```python
from build123d import *

# Parameters (mm, degrees)
F0_W      = 13
F0_H      = 7
F0_H_2    = 30.8050829545
F0_H_3    = 4
F1_DEPTH  = 13
F3_R      = 1.99999
F4_R      = 0.99999
F5_D      = 2.2
F7_W      = 3
F7_H      = 6.5
F6_W      = 66.7
F6_H      = 6.5
F8_DEPTH  = 2
F9_DEPTH  = 2
F10_R     = 3.5
F10_R_2   = 1.1
F11_DEPTH = 0.75


# Not quite as in the source:
# - a fillet or chamfer is up to 0.001 mm smaller than in the source, because OpenCascade refuses the exact size


with BuildPart() as f1:
    # F0 (on Top) → F1 (new body)
    with BuildSketch(Plane.XY):
        Polygon((-22, 0), (0, 0), (0, 3), (-19.5, 3), (-19.5, 5.3), (0, 5.3), (0, 72), (-15.5, 72), (-15.5, 100), (-20, 100), (-20, 62), (-18, 62), (-18, 59), (-20, 59), (-20, 22.1949170455), (-18, 22.1949170455), (-18, 19.1949170455), (-20, 19.1949170455), (-20, 9.1949170455), (-22, 9.1949170455), align=None)
        with Locations((-11.5, 12.6949170455)):
            Rectangle(F0_W, F0_H, mode=Mode.SUBTRACT)
        with Locations((-11.5, 40.5974585228)):
            Rectangle(F0_W, F0_H_2, mode=Mode.SUBTRACT)
        with Locations((-11.5, 67)):
            Rectangle(F0_W, F0_H_3, mode=Mode.SUBTRACT)
    extrude(amount=F1_DEPTH)

    # F3 (radius 2 in the source; OpenCascade refuses exactly that, so slightly less here)
    f3_edges = [f1.edges().sort_by_distance(p)[0] for p in [
        (-22, 0, 6.5),
        (-18, 69, 6.5),
        (-18, 65, 6.5),
        (-5, 69, 6.5),
        (-5, 65, 6.5),
        (-18, 56, 6.5),
        (-5, 56, 6.5),
        (-18, 25.194917, 6.5),
        (-5, 25.194917, 6.5),
        (-18, 9.194917, 6.5),
        (-5, 9.194917, 6.5),
        (-5, 16.194917, 6.5),
        (-18, 16.194917, 6.5),
    ]]
    fillet(f3_edges, radius=F3_R)

    # F4 (radius 1 in the source; OpenCascade refuses exactly that, so slightly less here)
    f4_edges = [f1.edges().sort_by_distance(p)[0] for p in [
        (-15.5, 72, 6.5),
        (-20, 100, 6.5),
        (-22, 9.194917, 6.5),
        (-20, 9.194917, 6.5),
    ]]
    fillet(f4_edges, radius=F4_R)

    # F5 (through all)
    with Locations(Plane(origin=(-20, 0, 0), x_dir=(0, -1, 0), z_dir=(-1, 0, 0))):
        with Locations((-90, 6.5)):
            Hole(F5_D / 2)

    # F7 (on face) + F6 (on face) → F8 (join)
    with BuildSketch(Plane.YZ):
        with Locations((1.5, 3.25)):
            Rectangle(F7_W, F7_H)
    with BuildSketch(Plane.YZ):
        with Locations((38.65, 3.25)):
            Rectangle(F6_W, F6_H)
    extrude(amount=F8_DEPTH)

    # F9 (cut): faces of the model
    f9_faces = [f1.faces().sort_by_distance(p)[0] for p in [
        (0, 1.5, 9.75),
        (0, 38.65, 9.75),
    ]]
    extrude(f9_faces, amount=-F9_DEPTH, mode=Mode.SUBTRACT)

    # F10 (on face) → F11 (cut)
    with BuildSketch(Plane.YZ.offset(-15.5)):
        with Locations((90, 6.5)):
            Circle(F10_R)
        with Locations((90, 6.5)):
            Circle(F10_R_2, mode=Mode.SUBTRACT)
    extrude(amount=-F11_DEPTH, mode=Mode.SUBTRACT)


solid = f1.part
```
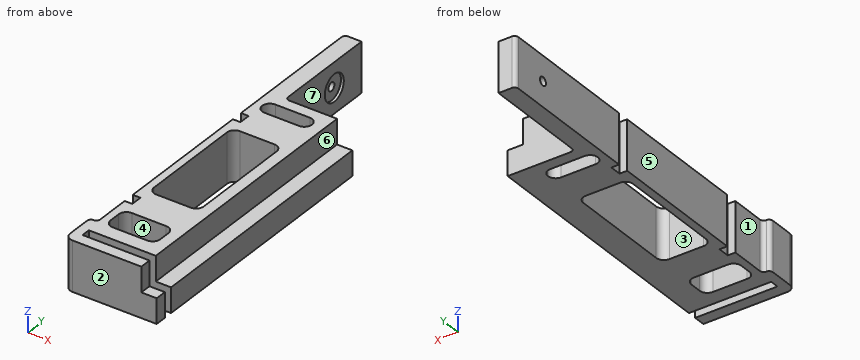
Geometry check sheet. Reference: the model listing, model coordinates, mm. Face numbers are marked on the shaded views. A direction names the side the tool comes from. Coordinates: 2 decimals unless noted, no trailing zeros. Order: outer loops, then holes, each group sorted by start corner. A loop starts at its lowest first (then second) coordinate and runs counter-clockwise, first axis right, second up. Notation, with made-up numbers: (13, -39) - (45, -39) arc R19 cw to (45, -13) - close; hole circle Ø1 at (-35, 5). An arc over 180 degrees is marked (long way). Use one line per item in the form item = value.
1. Access from +Z, -Z, +X, -X, +Y, -Y to the whole of each face (thin tool, end or side, straight path). Record for the marked faces 4, 5, 6 and 7.
Here are the results:
face_4 = +Z, -Z
face_5 = +Z, -Z, -X, +Y
face_6 = +Z, +X, +Y, -Y
face_7 = +Z, -Z, +X, +Y
2. Gauge pin test, flat ends, axial feed: pin 1 (1.5 mm diameter, centred on x = -16.5, y = 14, fed in from -Z); pin 2 (1 mm diameter, centred on x = -1, y = 55.5, fed in from -Z); pin 3 (6 mm diameter, centred on x = -0.5, z = 11, fed in from +Y); pin 4 (1.5 mm diameter, centred on y = 13, z = 4, fed in from -X). Record the tip position at first contact, or that the pin passes through.
Here are the results:
pin_1 = through
pin_2 = 0
pin_3 = 72
pin_4 = -20
3. Scan lines: line 1 (X direction, y = 52, z = 10.25); line 2 (Z direction, x = -15.75, y = 90); line 3 (Z direction, x = -17.35, y = 90). Record each from-to range of solid material in increasing order.
Here are the results:
line_1 = -20 to -18, -5 to -2
line_2 = 0 to 3, 10 to 13
line_3 = 0 to 5.4, 7.6 to 13
4. Section check A-A (x = -13.25). Record the boundary of the cut face in (y, z).
Here are the results:
outline = (0, 0) - (3, 0) - (3, 13) - (0, 13) - close; (5.3, 0) - (9.19, 0) - (9.19, 13) - (5.3, 13) - close; (16.19, 0) - (25.19, 0) - (25.19, 13) - (16.19, 13) - close; (56, 0) - (65, 0) - (65, 13) - (56, 13) - close; (69, 0) - (72, 0) - (72, 13) - (69, 13) - close
5. Section check D-D (y = 40). Record the boundary of the cut face in (x, z), then the cut area to 3 significant figures.
Here are the results:
outline = (-20, 0) - (-18, 0) - (-18, 13) - (-20, 13) - close; (-5, 0) - (2, 0) - (2, 6.5) - (-2, 6.5) - (-2, 13) - (-5, 13) - close
area = 91.0 mm²
6. Section check B-B (y = 90). Record the boundary of the cut face in (x, z), then the cut area to 3 significant figures.
Here are the results:
outline = (-20, 0) - (-15.5, 0) - (-15.5, 3) - (-16.25, 3) - (-16.25, 5.4) - (-20, 5.4) - close; (-20, 7.6) - (-16.25, 7.6) - (-16.25, 10) - (-15.5, 10) - (-15.5, 13) - (-20, 13) - close
area = 45.0 mm²
7. Draft check along Y on the marked faces 1, 2 and 3. Enter one of: pulls with the +Y half, pulls with the -Y half, needs draft (parallel to the pull), parting line crosses it, or undercut.
Here are the results:
face_1 = needs draft
face_2 = pulls with the -Y half
face_3 = undercut
8. Section check C-C (x = -4). Record the boundary of the cut face in (y, z), then the cut area to 3 significant figures.
Here are the results:
outline = (0, 0) - (3, 0) - (3, 13) - (0, 13) - close; (5.3, 0) - (72, 0) - (72, 13) - (5.3, 13) - close
area = 906 mm²
